Autodesk Inventor part; units mm, degrees
ref_plane "YZ Plane" through (0, 0, 0) normal (1, 0, 0) x (0, 1, 0)
ref_plane "XZ Plane" through (0, 0, 0) normal (0, 1, 0) x (-1, 0, 0)
ref_plane "XY Plane" through (0, 0, 0) normal (0, 0, 1) x (1, 0, 0)
sketch "Sketch1" plane through (0, 0, 0) normal (0, 0, 1) x (1, 0, 0)
  line L0 (-19.6117, 15.4854) -> (2.3883, 15.4854)
  line L1 (2.3883, 15.4854) -> (2.3883, 5.9854)
  line L2 (2.3883, 5.9854) -> (-19.6117, 5.9854)
  line L3 (-19.6117, 5.9854) -> (-19.6117, 15.4854)
  circle A0 centre (-17.6117, 10.7354) radius 1
  circle A1 centre (0.3883, 10.7354) radius 1
  point P0 (2.3883, 10.7354)
  dimension "d0" = 22
  dimension "d1" = 9.5
  dimension "d2" = 18
  dimension "d3" = 2
  dimension "d4" = 2
extrude "Extrusion1" add sketch "Sketch1" along normal blind 3
sketch "Sketch2" plane through (0, 0, 3) normal (0, 0, 1) x (1, 0, 0)
  line L0 (-19.6117, 15.4854) -> (2.3883, 15.4854)
  line L1 (-19.6117, 5.9854) -> (-19.6117, 15.4854)
  line L2 (2.3883, 5.9854) -> (-19.6117, 5.9854)
  line L3 (-15.0117, 15.4854) -> (-2.2117, 15.4854)
  line L4 (-2.2117, 15.4854) -> (-2.2117, 5.9854)
  line L5 (-2.2117, 5.9854) -> (-15.0117, 5.9854)
  line L6 (-15.0117, 5.9854) -> (-15.0117, 15.4854)
  point P0 (0, 0)
  point P1 (-8.6117, 5.9854)
  point P2 (-8.6117, 5.9854)
  dimension "d7" = 12.8
extrude "Extrusion2" add sketch "Sketch2" along normal blind 12 contours L0 L4 L2 L6
sketch "Sketch3" plane through (0, 0, 0) normal (0, 0, -1) x (-1, 0, 0)
  line L0 (19.6117, 15.4854) -> (-2.3883, 15.4854)
  line L1 (-2.3883, 5.9854) -> (19.6117, 5.9854)
  line L2 (15.0117, 5.9854) -> (2.2117, 5.9854)
  line L3 (2.2117, 5.9854) -> (2.2117, 15.4854)
  line L4 (2.2117, 15.4854) -> (15.0117, 15.4854)
  line L5 (15.0117, 15.4854) -> (15.0117, 5.9854)
  point P0 (0, 0)
  point P1 (8.6117, 5.9854)
  point P2 (8.6117, 5.9854)
  dimension "d10" = 12.8
extrude "Extrusion3" add sketch "Sketch3" along normal blind 12
sketch "Sketch4" plane through (0, 0, -12) normal (0, 0, -1) x (-1, 0, 0)
  line L0 (2.2117, 5.9854) -> (2.2117, 15.4854)
  line L1 (15.0117, 5.9854) -> (2.2117, 5.9854)
  line L2 (13.6117, 6.9354) -> (3.6117, 6.9354)
  line L3 (3.6117, 6.9354) -> (3.6117, 14.5354)
  line L4 (3.6117, 14.5354) -> (13.6117, 14.5354)
  line L5 (13.6117, 14.5354) -> (13.6117, 6.9354)
  point P0 (0, 0)
  point P1 (8.6117, 5.9854)
  point P2 (8.6117, 6.9354)
  point P3 (3.6117, 10.7354)
  point P4 (2.2117, 10.7354)
  dimension "d13" = 10
  dimension "d14" = 7.6
extrude "Extrusion4" cut sketch "Sketch4" against normal blind 30
sketch "Sketch5" plane through (-19.6117, 5.9854, 0) normal (0, -1, 0) x (1, 0, 0)
  line L0 (17.4, 15) -> (4.6, 15)
  line L1 (4.6, 3) -> (4.6, 15)
  line L2 (4.6, 0) -> (4.6, -12)
  line L3 (4.6, -12) -> (17.4, -12)
  arc A0 (10, 8) -> (12, 8) centre (11, 8) ccw
  arc A1 (12, -5) -> (10, -5) centre (11, -5) ccw
  line L4 (10, 8) -> (10, 15)
  line L5 (12, 8) -> (12, 15)
  line L6 (10, -5) -> (10, -12)
  line L7 (12, -5) -> (12, -12)
  point P0 (19.6117, 0)
  point P1 (11, 15)
  dimension "d17" = 7
  dimension "d18" = 7
  dimension "d19" = 2
extrude "Extrusion5" cut sketch "Sketch5" against normal blind 3
properties part number "SC-adapter" material "ABS Plastic"
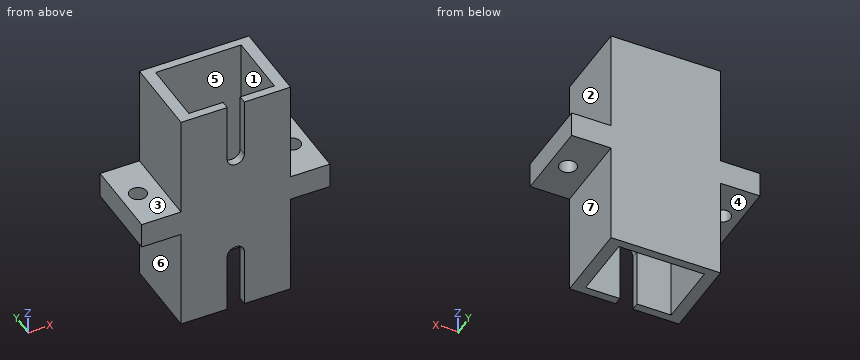
Part model, mm, in its own coordinate system. Face numbers are marked on the shaded views. A direction names the side the tool comes from. Give positions to 0.01 mm unless a question says otherwise; leave off trailing zeros. Write each loop counter-clockwise with the first axis right and the second up, starting at its lowest first coordinate (ties: lowest second). Pieces come first, ordered by that corner, then holes. Notation, with made-up numbers: M 77.5,-37 L 99.5,-37 A23 ccw 99.5,-27 Z; hole C 60.25,50 d9. An arc over 180 degrees is marked long. Use CSV: the item, a comma, the result in double quotes.
Item 1: Which spindle directions (+Z, -Z, +X, -X, +Y, -Y) get a long thin tool onto all of the face, cutting with end or side? Do the marked faces 1, 2 and 3. Say none if no direction does.
Taken from the geometry:
face 1,"+Z, -Z"
face 2,"+Z, +X, +Y, -Y"
face 3,"+Z, -X, +Y, -Y"
Item 2: Slice it at B-B on y = 9. Write the cut outline in (x, z).
Taken from the geometry:
outline,"M -19.61,0 L -15.01,0 L -15.01,-12 L -13.61,-12 L -13.61,15 L -15.01,15 L -15.01,3 L -19.61,3 Z; M -3.61,-12 L -2.21,-12 L -2.21,0 L 2.39,0 L 2.39,3 L -2.21,3 L -2.21,15 L -3.61,15 Z"
Item 3: Drill centre lines: probe 1 along Y at (x, z) = (-8.75, 3); probe 2 along X at (y, z) = (11.25, -0.25); probe 3 along X at (y, z) = (9.25, 2.5). Where is each one in solid material? Low to high.
Taken from the geometry:
probe 1,"y = 5.99 to 6.94, 14.54 to 15.49"
probe 2,"x = -15.01 to -13.61, -3.61 to -2.21"
probe 3,"x = -19.61 to -13.61, -3.61 to 2.39"
Item 4: Slice it at D-D on x = 0. Write the cut outline in (y, z), plus the area to 3 significant figures.
Taken from the geometry:
outline,"M 5.99,0 L 9.81,0 L 9.81,3 L 5.99,3 Z; M 11.66,0 L 15.49,0 L 15.49,3 L 11.66,3 Z"
area,"23.0 mm²"
Item 5: Slice it at C-C on z = 9.5. Write the cut outline in (x, y), plus the area to 3 significant figures.
Taken from the geometry:
outline,"M -15.01,5.99 L -9.61,5.99 L -9.61,6.94 L -13.61,6.94 L -13.61,14.54 L -3.61,14.54 L -3.61,6.94 L -7.61,6.94 L -7.61,5.99 L -2.21,5.99 L -2.21,15.49 L -15.01,15.49 Z"
area,"43.7 mm²"
Item 6: Slice it at A-A on x = -10.5. Write the cut outline in (y, z), plus the area to 3 significant figures.
Taken from the geometry:
outline,"M 5.99,-12 L 6.94,-12 L 6.94,15 L 5.99,15 Z; M 14.54,-12 L 15.49,-12 L 15.49,15 L 14.54,15 Z"
area,"51.3 mm²"
Item 7: Pull direction X, two halves, no side cores. Call the marked faces 4, 5, 6 and 7: +X half, -X half, draft (parallel to the pull), parting line (faces both ways), or undercut.
Taken from the geometry:
face 4,"draft"
face 5,"undercut"
face 6,"-X half"
face 7,"+X half"
Item 8: Pin check, flat tips, straight feed: P1, Ø5, axis at x = 1, y = 11, coming from the +Z side; P2, Ø0.5, axis at y = 6.5, z = -9.5, coming from the -X side; P3, Ø1.5, axis at x = -8.5, y = 14, coming from the -Z side; P4, Ø1, axis at y = 6.5, z = 10.5, coming from the +X side. Stop position of each tip, or through.
Taken from the geometry:
P1,"stops at z = 3"
P2,"stops at x = -15.01"
P3,"stops at z = -12"
P4,"stops at x = -2.21"
